```python
from build123d import *

# Parameters (mm, degrees)
F0_W        = 110
F0_H        = 50
F1_DEPTH    = 16
F2_SIZE     = 15.99999
F3_T1_DEPTH = 192.2938556149


# Not quite as in the source:
# - a fillet or chamfer that OpenCascade refuses, or shapes differently, is made with other operations: its cross-section is extruded or revolved along the edge and cut away or added
# - a fillet or chamfer is up to 0.001 mm smaller than in the source, because OpenCascade refuses the exact size


with BuildPart() as f1:
    # F0 (on Top) → F1 (new body)
    with BuildSketch(Plane.XY):
        with Locations((55, 25)):
            Rectangle(F0_W, F0_H)
        Polygon((17.5, 36.5), (55, 36.5), (92.5, 36.5), (92.5, 27.5), (17.5, 27.5), align=None, mode=Mode.SUBTRACT)
    extrude(amount=F1_DEPTH)

    # F2 (size 16 in the source; OpenCascade refuses exactly that, so slightly less here)
    f2_edges = [f1.edges().sort_by_distance(p)[0] for p in [
        (55, 0, 16),
    ]]
    chamfer(f2_edges, length=F2_SIZE)

    # F3: chamfer of 16 on 1 edges, made by hand

    # F3_s2 → F3_t1 (cut)
    with BuildSketch(Plane.YZ.offset(-41.1469278075)):
        Polygon((34, 0), (50, 16), (50, 0), align=None)
    extrude(amount=F3_T1_DEPTH, mode=Mode.SUBTRACT)


solid = f1.part
```
Geometry check sheet. Reference: the model listing, model coordinates, mm. A direction names the side the tool comes from. Coordinates: 2 decimals unless noted, no trailing zeros. Loops run counter-clockwise (first coordinate to the right, second up) from the corner with the lowest first, then second, coordinate; pieces in that order, holes last. Notation, with made-up numbers: (-1.5, -7.5) - (39.5, -7.5) arc R10 cw to (39.5, -0.5) - close; hole circle Ø3 at (48.5, -7). An arc over 180 degrees is marked (long way). One line per item, written item: value. Start each with the question number.
(1) Depth check by flat-ended pin: P1, Ø1.5, axis at y = 41, z = 5.5, coming from the -X side; P2, Ø4, axis at x = 42, z = 12, coming from the -Y side; P3, Ø4, axis at x = 70, z = 5, coming from the +Y side; P4, Ø3, axis at x = 45.5, z = 7.5, coming from the -Y side. Enter the tip coordinate at first touch or a pass-through.
(2) Cross-section at B-B on z = 10. Enter the section's corners in (x, y).
(3) Material ranges on line 1 (X direction, y = 36, z = 4.75); line 2 (Y direction, x = 87, z = 7.75); line 3 (Y direction, x = 40.5, z = 15), recorded low to high. Write a range as [from, to].
(4) Tool access check on faces 1 (the flat face through (54, 37, 16)), 2 (the flat face through (17.5, 32, 8)). Record the directions out of +Z, -Z, +X, -X, +Y, -Y that give a thin tool (end or side, any length) a straight path to the whole face; none if there is none.
(5) Cross-section at C-C on y = 44.5. Enter the section's corners in (x, z), plus the area to 3 significant figures.
(6) Cross-section at D-D on z = 1.5. Enter the section's corners in (x, y).
(7) Mould release check, pull along Y, two halves, no side actions. Record for faces 3 (the flat face through (54, 8, 8)), 4 (the flat face through (54, 42, 8)), 5 (the flat face through (56, 27.5, 8)), 6 (the flat face through (54, 13, 0)): released by +Y, released by -Y, zero draft, split by the parting line, or undercut.
Results below:
1. P1: passes through
1. P2: stops at y = 10
1. P3: stops at y = 41
1. P4: stops at y = 6
2. outline: (0, 10) - (110, 10) - (110, 44) - (0, 44) - close; hole (17.5, 27.5) - (92.5, 27.5) - (92.5, 36.5) - (17.5, 36.5) - close
3. line 1: x = [0, 17.5], [92.5, 110]
3. line 2: y = [7.75, 27.5], [36.5, 41.75]
3. line 3: y = [15, 27.5], [36.5, 49]
4. face 1: +Z, +X, -X, +Y, -Y
4. face 2: +Z, -Z
5. outline: (0, 10.5) - (110, 10.5) - (110, 16) - (0, 16) - close
5. area: 605 mm2
6. outline: (0, 1.5) - (110, 1.5) - (110, 35.5) - (92.5, 35.5) - (92.5, 27.5) - (17.5, 27.5) - (17.5, 35.5) - (0, 35.5) - close
7. face 3: released by -Y
7. face 4: released by +Y
7. face 5: undercut
7. face 6: zero draft
